For this review, take the finished solid that the model builds, in its own axes (mm). Face numbers are marked on the shaded views. A direction names the side the tool comes from. Give positions to 0.01 mm unless a question says otherwise; leave off trailing zeros. Write each loop counter-clockwise with the first axis right and the second up, starting at its lowest first coordinate (ties: lowest second). Pieces come first, ordered by that corner, then holes. Notation, with made-up numbers: M 54.25,81.25 L 100.25,81.25 A25 ccw 100.25,95.25 Z; hole C 87,60 d8. An arc over 180 degrees is marked long. Answer as a JSON object with one key per item and string values. Group by question number.
```python
from build123d import *

# Parameters (mm, degrees)
F0_W     = 133.35
F0_H     = 101.6
F1_DEPTH = 19.05
F2_T     = -3.175
F3_R     = 6.35
F4_DEPTH = 3.175
F5_R     = 3.175
F6_DEPTH = 12.7
F7_R     = 3.175
F8_DEPTH = 12.7
F9_R     = 6.35
F10_SIZE = 1.6002


with BuildPart() as f1:
    # F0 (on Front) → F1 (new body)
    with BuildSketch(Plane.XZ):
        with Locations((66.675, -50.8)):
            Rectangle(F0_W, F0_H)
    extrude(amount=F1_DEPTH)

    # F2
    f2_openings = [f1.faces().sort_by_distance(p)[0] for p in [
        (66.675, -19.05, -50.8),
    ]]
    offset(amount=F2_T, openings=f2_openings)

    # F3 (on face) → F4 (join)
    with BuildSketch(Plane.XZ.offset(3.175)):
        with Locations((28.575, -50.8)):
            Circle(F3_R)
        with Locations((85.725, -50.8)):
            Circle(F3_R)
    extrude(amount=F4_DEPTH)

    # F5 (on face) → F6 (join)
    with BuildSketch(Plane.XZ.offset(6.35)):
        with Locations((28.575, -50.8)):
            Circle(F5_R)
    extrude(amount=F6_DEPTH)

    # F7 (on face) → F8 (join)
    with BuildSketch(Plane.XZ.offset(6.35)):
        with Locations((85.725, -50.8)):
            Circle(F7_R)
    extrude(amount=F8_DEPTH)

    # F9
    f9_edges = [f1.edges().sort_by_distance(p)[0] for p in [
        (3.175, -11.1125, -3.175),
        (130.175, -11.1125, -3.175),
        (3.175, -11.1125, -98.425),
        (130.175, -11.1125, -98.425),
    ]]
    fillet(f9_edges, radius=F9_R)

    # F10
    f10_edges = [f1.edges().sort_by_distance(p)[0] for p in [
        (66.675, -19.05, -101.6),
        (133.35, -19.05, -50.8),
        (66.675, -19.05, 0),
        (0, -19.05, -50.8),
    ]]
    chamfer(f10_edges, length=F10_SIZE)


solid = f1.part
```
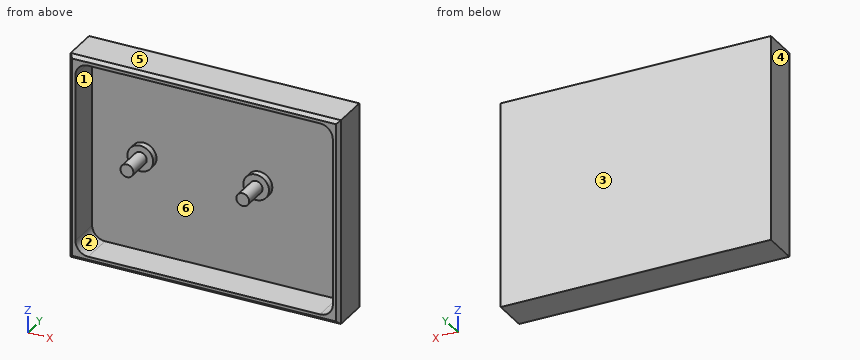
Item 1: Machinability: for the marked faces 5 and 6, which of the approach directions +Z, -Z, +X, -X, +Y, -Y give a long, thin tool a straight path to every point of the face, cutting with its end or side? Answer none if there is none.
Item 2: Consider section C-C (z = -70). Give the boundary of the cut face in (x, y) (3 decimals), plus the area to 3 significant figures.
Item 3: Insertion check: P1, Ø3, axis at x = 37, z = -65.5, coming from the -Y side (3 decimals). The pin has a flat end and moves straight along its axis. Give the tip position at first contact, or say it passes through.
Item 4: Draft analysis for pull direction X (two halves, no side actions). For the marked faces 1, 2, 3 and 4, state which applies: released by +X, released by -X, zero draft, split by the parting line, or undercut.
Item 5: Consider section D-D (y = -4.75). Give the boundary of the cut face in (x, z) (3 decimals), plus the area to 3 significant figures.
Item 6: Consider section A-A (y = -11.75). Give the boundary of the cut face in (x, z) (3 decimals).
Item 7: To check wall thickness, follow probe 1 along X at (y, z) = (-3.5, -51) (3 decimals); probe 2 along X at (y, z) = (-4.5, -13.5) (3 decimals); probe 3 along Z at (x, y) = (64, -15.75) (3 decimals). State the ranges of each line that lie inside material, in increasing order.
Item 8: Consider section B-B (x = 11.5). Give the boundary of the cut face in (y, z) (3 decimals).
Result set:
{
 "1": {"face 5": "+Z, +X, -X, +Y, -Y", "face 6": "-Y"},
 "2": {"outline": "M 0,-17.45 L 1.6,-19.05 L 3.175,-19.05 L 3.175,-3.175 L 130.175,-3.175 L 130.175,-19.05 L 131.75,-19.05 L 133.35,-17.45 L 133.35,0 L 0,0 Z", "area": "522 mm^2"},
 "3": {"P1": "stops at y = -3.175"},
 "4": {"face 1": "undercut", "face 2": "undercut", "face 3": "zero draft", "face 4": "released by -X"},
 "5": {"outline": "M 0,-101.6 L 133.35,-101.6 L 133.35,0 L 0,0 Z; C 28.575,-50.8 d12.7; C 85.725,-50.8 d12.7; hole M 3.175,-92.075 A6.35 ccw 9.525,-98.425 L 123.825,-98.425 A6.35 ccw 130.175,-92.075 L 130.175,-9.525 A6.35 ccw 123.825,-3.175 L 9.525,-3.175 A6.35 ccw 3.175,-9.525 Z", "area": "1,740 mm^2"},
 "6": {"outline": "M 0,-101.6 L 133.35,-101.6 L 133.35,0 L 0,0 Z; C 28.575,-50.8 d6.35; C 85.725,-50.8 d6.35; hole M 3.175,-92.075 A6.35 ccw 9.525,-98.425 L 123.825,-98.425 A6.35 ccw 130.175,-92.075 L 130.175,-9.525 A6.35 ccw 123.825,-3.175 L 9.525,-3.175 A6.35 ccw 3.175,-9.525 Z"},
 "7": {"probe 1": "x = 0 to 3.175, 22.228 to 34.922, 79.378 to 92.072, 130.175 to 133.35", "probe 2": "x = 0 to 3.175, 130.175 to 133.35", "probe 3": "z = -101.6 to -98.425, -3.175 to 0"},
 "8": {"outline": "M -19.05,-100 L -17.45,-101.6 L 0,-101.6 L 0,0 L -17.45,0 L -19.05,-1.6 L -19.05,-3.175 L -3.175,-3.175 L -3.175,-98.425 L -19.05,-98.425 Z"}
}
